Check sheet for the drawn part. Datum: minimum x, y, z corner. Units: mm. A direction names the side the tool comes from. Coordinates: 2 decimals unless noted, no trailing zeros. Loops run counter-clockwise (first coordinate to the right, second up) from the corner with the lowest first, then second, coordinate; pieces in that order, holes last. Notation, with made-up numbers: (-38, 88.25) -> (-23, 88.25) arc R36 cw to (-23, 124.25) -> close; hole circle Ø8 at (23, 48). An arc over 180 degrees is marked (long way). Use CSV: the item, a comma, the result in double quotes. Start each with the question number.
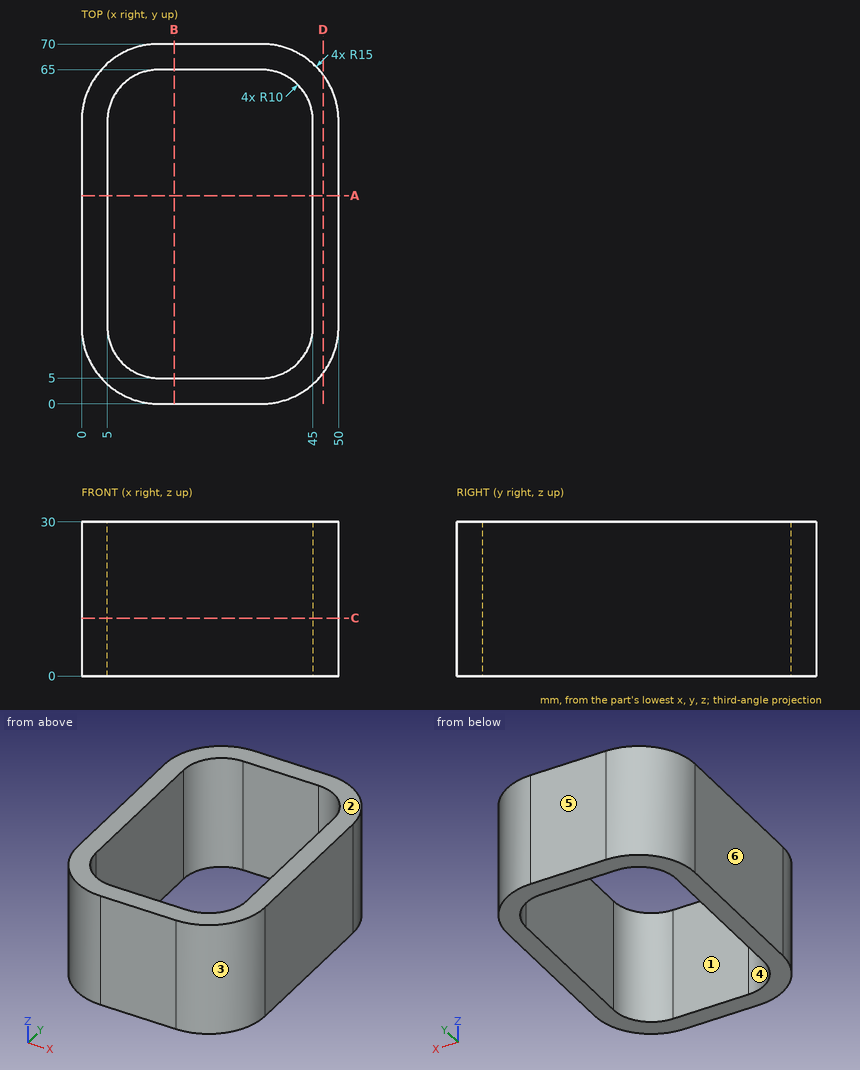
1. Set-up check for the marked faces 1 and 2: record each of +Z, -Z, +X, -X, +Y, -Y from which the full face is reachable in a straight line by a thin tool's end or side.
2. Depth check by flat-ended pin: pin 1 (6 mm diameter, centred on x = 40, y = 42, fed in from +Z); pin 2 (1.5 mm diameter, centred on y = 58, z = 26, fed in from +X). Enter the tip coordinate at first touch or a pass-through.
3. Cross-section at B-B, the plane x = 18. Record the boundary of the cut face in (y, z).
4. Cross-section at C-C, the plane z = 11.25. Record the boundary of the cut face in (x, y).
5. Release check for a two-part mould opening along Y. For the marked faces 3, 4, 5 and 6 record: released by +Y, released by -Y, zero draft, split by the parting line, or undercut.
6. Cross-section at D-D, the plane x = 47. Record the boundary of the cut face in (y, z), plus the area to 3 significant figures.
7. Scan lines: line 1 (Y direction, x = 29, z = 23); line 2 (X direction, y = 22, z = 23); line 3 (X direction, y = 62.5, z = 16.75). Record each from-to range of solid material in increasing order.
8. Cross-section at A-A, the plane y = 40.5. Record the boundary of the cut face in (x, z).
Solution:
1,face 1,"+Z, -Z"
1,face 2,"+Z, +X, -X, +Y, -Y"
2,pin 1,"passes through"
2,pin 2,"stops at x = 49.83"
3,outline,"(0, 0) -> (5, 0) -> (5, 30) -> (0, 30) -> close; (65, 0) -> (70, 0) -> (70, 30) -> (65, 30) -> close"
4,outline,"(0, 15) arc R15 ccw to (15, 0) -> (35, 0) arc R15 ccw to (50, 15) -> (50, 55) arc R15 ccw to (35, 70) -> (15, 70) arc R15 ccw to (0, 55) -> close; hole (5, 15) arc R10 ccw to (15, 5) -> (35, 5) arc R10 ccw to (45, 15) -> (45, 55) arc R10 ccw to (35, 65) -> (15, 65) arc R10 ccw to (5, 55) -> close"
5,face 3,"released by -Y"
5,face 4,"undercut"
5,face 5,"released by +Y"
5,face 6,"zero draft"
6,outline,"(6, 0) -> (64, 0) -> (64, 30) -> (6, 30) -> close"
6,area,"1,740 mm2"
7,line 1,"y = 0 to 5, 65 to 70"
7,line 2,"x = 0 to 5, 45 to 50"
7,line 3,"x = 2.01 to 8.39, 41.61 to 47.99"
8,outline,"(0, 0) -> (5, 0) -> (5, 30) -> (0, 30) -> close; (45, 0) -> (50, 0) -> (50, 30) -> (45, 30) -> close"
